from build123d import *

# Parameters (mm, degrees)
EXTRUDE_1_OUTLINE_R   = 100
EXTRUDE_1_OUTLINE_R_2 = 3
EXTRUDE_1_OUTLINE_W   = 42
EXTRUDE_1_OUTLINE_H   = 42
EXTRUDE_1_DEPTH       = 3
SKETCH_2_R            = 13
SKETCH_2_R_2          = 2
CUT_EXTRUDE_1_DEPTH   = 3


# Read off the part's stored shape, not the designer's step: Бобышка-Вытянуть1
with BuildPart() as part:
    # Бобышка-Вытянуть1 outline → Бобышка-Вытянуть1 (new body)
    with BuildSketch(Plane(origin=(0, 0, 0), x_dir=(1, 0, 0), z_dir=(0, 1, 0))):
        Circle(EXTRUDE_1_OUTLINE_R)
        with Locations((-67.175120484, -67.175120484)):
            Circle(EXTRUDE_1_OUTLINE_R_2, mode=Mode.SUBTRACT)
        with Locations((0, -95)):
            Circle(EXTRUDE_1_OUTLINE_R_2, mode=Mode.SUBTRACT)
        with Locations((67.175120484, -67.175120484)):
            Circle(EXTRUDE_1_OUTLINE_R_2, mode=Mode.SUBTRACT)
        with Locations((-95, 0)):
            Circle(EXTRUDE_1_OUTLINE_R_2, mode=Mode.SUBTRACT)
        with Locations((-67.175120484, 67.175120484)):
            Circle(EXTRUDE_1_OUTLINE_R_2, mode=Mode.SUBTRACT)
        Rectangle(EXTRUDE_1_OUTLINE_W, EXTRUDE_1_OUTLINE_H, mode=Mode.SUBTRACT)
        with Locations((95, 0)):
            Circle(EXTRUDE_1_OUTLINE_R_2, mode=Mode.SUBTRACT)
        with Locations((0, 95)):
            Circle(EXTRUDE_1_OUTLINE_R_2, mode=Mode.SUBTRACT)
        with Locations((67.175120484, 67.175120484)):
            Circle(EXTRUDE_1_OUTLINE_R_2, mode=Mode.SUBTRACT)
    extrude(amount=EXTRUDE_1_DEPTH)

    # Эскиз2 → Вырез-Вытянуть1 (cut)
    with BuildSketch(Plane(origin=(0, 3, 0), x_dir=(1, 0, 0), z_dir=(0, 1, 0))):
        with Locations(Location((0, 54.663461451, 0), (0, 0, 270))):
            Circle(SKETCH_2_R)
        with Locations(Location((25, 0, 0), (0, 0, 270))):
            Circle(SKETCH_2_R_2)
        with Locations(Location((0, 25, 0), (0, 0, 270))):
            Circle(SKETCH_2_R_2)
        with Locations(Location((-25, 0, 0), (0, 0, 270))):
            Circle(SKETCH_2_R_2)
        with Locations(Location((0, -25, 0), (0, 0, 270))):
            Circle(SKETCH_2_R_2)
    extrude(amount=-CUT_EXTRUDE_1_DEPTH, mode=Mode.SUBTRACT)


solid = part.part
Verification items for the finished model (mm, model axes). Round coordinates to 2 decimals unless told otherwise and drop trailing zeros. Order: outer loops, then holes, each group sorted by start corner. A loop starts at its lowest first (then second) coordinate and runs counter-clockwise, first axis right, second up.
1. Thickness scan on L1, parallel to X at y = 2.45, z = 0; L2, parallel to Z at x = 66.5, y = 0.6; L3, parallel to Z at x = -26.5, y = 2.75. Record the ranges inside material, lowest first.
Final values:
L1: x = -100 to -98, -92 to -27, -23 to -21, 21 to 23, 27 to 92, 98 to 100
L2: z = -74.68 to -70.1, -64.25 to 64.25, 70.1 to 74.68
L3: z = -96.42 to -1.32, 1.32 to 96.42
2. Go/stop test with flat-tipped pins: P1, Ø1.5, axis at x = -16.5, y = 1, coming from the +Z side; P2, Ø0.9, axis at x = -8.5, y = 1.5, coming from the +Z side; P3, Ø1, axis at y = 2, z = -73, coming from the +X side. Record where each tip stops, or that it passes through.
Final values:
P1: stops at z = 98.75
P2: stops at z = 99.68
P3: stops at x = 68.87
3. Section check D-D on z = 84. Record the cut outline in (x, y), then the cut area to 3 significant figures.
Final values:
outline: (-54.26, 0) - (54.26, 0) - (54.26, 3) - (-54.26, 3) - close
area: 326 mm2
4. Section check C-C on y = 2. State how many separate pieces and enclosed holes the cut face has, then the cut area to 3 significant figures.
Final values:
separate pieces: 1
enclosed holes: 14
area: 28,800 mm2
5. Release check for a two-part mould opening along X. For faces 1 (the cylindrical face through (68.559, 1.479, -64.514)), 2 (the cylindrical face through (95.38, 1.48, -30.04)), 3 (the flat face through (-24, 3, 21)), 4 (the cylindrical face through (-69.556, 1.479, -65.35)) record: +X half, -X half, draft (parallel to the pull), parting line (faces both ways), or undercut.
Final values:
face 1: undercut
face 2: parting line
face 3: draft
face 4: undercut
6. Section check B-B on z = 11. Record the cut outline in (x, y).
Final values:
outline: (-99.39, 0) - (-21, 0) - (-21, 3) - (-99.39, 3) - close; (21, 0) - (99.39, 0) - (99.39, 3) - (21, 3) - close
7. Section check A-A on x = -95. Record the cut outline in (y, z).
Final values:
outline: (0, -31.22) - (3, -31.22) - (3, -3) - (0, -3) - close; (0, 3) - (3, 3) - (3, 31.22) - (0, 31.22) - close
